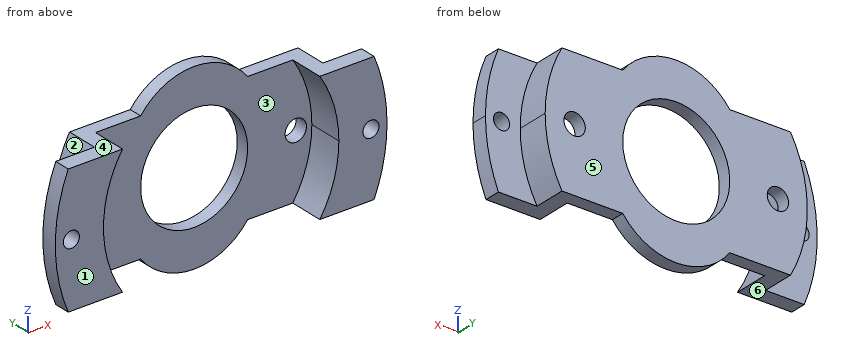
from build123d import *

# Parameters (mm, degrees)
F0_R     = 2
F0_R_2   = 10
F1_DEPTH = 2.5
F2_DEPTH = 9
F3_R     = 1.5
F4_DEPTH = 3
F5_DEPTH = 2.5


with BuildPart() as f1:
    # F0 (on Front) → F1 (new body)
    with BuildSketch(Plane.XZ):
        with BuildLine():
            ThreePointArc((22, 0), (21.090993, 6.258596), (18.439089, 12))
            Line((18.439089, 12), (10, 12))
            Line((10, 12), (-10, 12))
            Line((-10, 12), (-18.439089, 12))
            ThreePointArc((-18.439089, 12), (-22, 0), (-18.439089, -12))
            Line((-18.439089, -12), (-10, -12))
            Line((-10, -12), (10, -12))
            Line((10, -12), (18.439089, -12))
            ThreePointArc((18.439089, -12), (21.090993, -6.258596), (22, 0))
        make_face()
        with Locations((-19, 0)):
            Circle(F0_R, mode=Mode.SUBTRACT)
        Circle(F0_R_2, mode=Mode.SUBTRACT)
        with Locations((19, 0)):
            Circle(F0_R, mode=Mode.SUBTRACT)
    extrude(amount=F1_DEPTH)

    # F0 (on Front) → F2 (join)
    with BuildSketch(Plane.XZ):
        with BuildLine():
            ThreePointArc((24.5, 0), (23.702007, 6.202007), (21.360009, 12))
            Line((21.360009, 12), (18.439089, 12))
            ThreePointArc((18.439089, 12), (21.090993, 6.258596), (22, 0))
            ThreePointArc((22, 0), (21.090993, -6.258596), (18.439089, -12))
            Line((18.439089, -12), (21.360009, -12))
            ThreePointArc((21.360009, -12), (23.702007, -6.202007), (24.5, 0))
        make_face()
        with BuildLine():
            Line((-18.439089, 12), (-21.360009, 12))
            ThreePointArc((-21.360009, 12), (-24.5, 0), (-21.360009, -12))
            Line((-21.360009, -12), (-18.439089, -12))
            ThreePointArc((-18.439089, -12), (-22, 0), (-18.439089, 12))
        make_face()
    extrude(amount=F2_DEPTH)

    # F3 (on face) → F4 (join)
    with BuildSketch(Plane.XZ.offset(9)):
        with BuildLine():
            Line((-21.360009, 12), (-28.583212, 12))
            ThreePointArc((-28.583212, 12), (-31, 0), (-28.583212, -12))
            Line((-28.583212, -12), (-21.360009, -12))
            ThreePointArc((-21.360009, -12), (-24.5, 0), (-21.360009, 12))
        make_face()
        with Locations((-28, 0)):
            Circle(F3_R, mode=Mode.SUBTRACT)
        with BuildLine():
            ThreePointArc((28.583212, -12), (30.389797, -6.120475), (31, 0))
            ThreePointArc((31, 0), (30.389797, 6.120475), (28.583212, 12))
            Line((28.583212, 12), (21.360009, 12))
            ThreePointArc((21.360009, 12), (23.702007, 6.202007), (24.5, 0))
            ThreePointArc((24.5, 0), (23.702007, -6.202007), (21.360009, -12))
            Line((21.360009, -12), (28.583212, -12))
        make_face()
        with Locations((28, 0)):
            Circle(F3_R, mode=Mode.SUBTRACT)
    extrude(amount=-F4_DEPTH)

    # F0 (on Front) → F5 (join)
    with BuildSketch(Plane.XZ):
        with BuildLine():
            Line((-10, 12), (10, 12))
            ThreePointArc((10, 12), (0, 17), (-10, 12))
        make_face()
        with BuildLine():
            ThreePointArc((-10, -12), (0, -17), (10, -12))
            Line((10, -12), (-10, -12))
        make_face()
    extrude(amount=F5_DEPTH)


solid = f1.part
Check sheet for the modelled part. Datum: model origin and axes. Units: mm. Face numbers are marked on the shaded views. A direction names the side the tool comes from. Give positions to 0.01 mm unless a question says otherwise; leave off trailing zeros. Loops run counter-clockwise (first coordinate to the right, second up) from the corner with the lowest first, then second, coordinate; pieces in that order, holes last. Notation, with made-up numbers: M 67.5,85.25 L 102.5,85.25 A23 ccw 102.5,102.25 Z; hole C 64,49 d4. An arc over 180 degrees is marked long. Use a Markdown table: item, result. Add a question column.
Q1. Sectioned sample at D-D, the plane y = -0.75. Record the cut outline in (x, z), then the cut area to 3 significant figures.
Q2. Mould release check, pull along X, two halves, no side actions. Record for the marked faces 1, 2 and 3: pulls with the +X half, pulls with the -X half, needs draft (parallel to the pull), parting line crosses it, or undercut.
Q3. Sectioned sample at B-B, the plane y = -8. Record the cut outline in (x, z).
Q4. Sectioned sample at A-A, the plane y = -4.5. Record the cut outline in (x, z), then the cut area to 3 significant figures.
Q5. Scan lines: line 1 along Z through (x, y) = (-19, -0.9); line 2 along Z through (x, y) = (-28, -7.55); line 3 along X through (y, z) = (-7.5, 11). Record each from-to range of solid material in increasing order. Write a range as [from, to].
Q6. Sectioned sample at C-C, the plane x = 28. Record the cut outline in (y, z).
Q7. Tool access check on the marked faces 4, 5 and 6. Record the directions out of +Z, -Z, +X, -X, +Y, -Y that give a thin tool (end or side, any length) a straight path to the whole face; none if there is none.
Q8. Go/stop test with flat-tipped pins: pin 1 (10 mm diameter, centred on x = -1, z = -2, fed in from -Y); pin 2 (4.5 mm diameter, centred on x = -23.5, y = -4.5, fed in from +Z); pin 3 (7.5 mm diameter, centred on x = -28.5, z = -2.5, fed in from +Y); pin 4 (1 mm diameter, centred on y = -7.5, z = -3.5, fed in from +X). Record where each tip stops, or that it passes through.
Verdict:
| question | item | result |
|---|---|---|
| 1 | outline | M -21.36,-12 L -10,-12 A12.5 ccw 10,-12 L 21.36,-12 A24.5 ccw 24.5,0 A24.5 ccw 21.36,12 L 10,12 A12.5 ccw -10,12 L -21.36,12 A24.5 ccw Z; hole C -19,0 d4; hole C 0,0 d20; hole C 19,0 d4 |
| 1 | area | 928 mm^2 |
| 2 | face 1 | needs draft |
| 2 | face 2 | pulls with the -X half |
| 2 | face 3 | undercut |
| 3 | outline | M -28.58,-12 L -18.44,-12 A22 cw -18.44,12 L -28.58,12 A31 ccw Z; M 18.44,-12 L 28.58,-12 A31 ccw 31,0 A31 ccw 28.58,12 L 18.44,12 A22 cw 22,0 A22 cw Z; hole C -28,0 d3; hole C 28,0 d3 |
| 4 | outline | M -21.36,-12 L -18.44,-12 A22 cw -18.44,12 L -21.36,12 A24.5 ccw Z; M 18.44,-12 L 21.36,-12 A24.5 ccw 24.5,0 A24.5 ccw 21.36,12 L 18.44,12 A22 cw 22,0 A22 cw Z |
| 4 | area | 126 mm^2 |
| 5 | line 1 | [-12, -2], [2, 12] |
| 5 | line 2 | [-12, -1.5], [1.5, 12] |
| 5 | line 3 | [-28.98, -19.05], [19.05, 28.98] |
| 6 | outline | M -9,-12 L -6,-12 L -6,-1.5 L -9,-1.5 Z; M -9,1.5 L -6,1.5 L -6,12 L -9,12 Z |
| 7 | face 4 | +Z, -X, +Y, -Y |
| 7 | face 5 | +Z, -Z, +X, -X, +Y |
| 7 | face 6 | -Z, -X, +Y, -Y |
| 8 | pin 1 | through |
| 8 | pin 2 | z = 12 |
| 8 | pin 3 | y = -6 |
| 8 | pin 4 | x = 30.85 |
